```python
from build123d import *

# Parameters (mm, degrees)
F0_R      = 16.890202
F1_DEPTH  = 12.7
F2_R      = 12.7
F3_DEPTH  = 50.8
F5_R      = 16.890202
F6_DEPTH  = 12.7
F7_R      = 3.429
F8_DEPTH  = 12.701
F10_DEPTH = 12.7


with BuildPart() as f1:
    # F0 (on Front) → F1 (new body, symmetric)
    with BuildSketch(Plane.XZ):
        Circle(F0_R)
    extrude(amount=F1_DEPTH, both=True)

    # F2 (on Top) → F3 (join)
    with BuildSketch(Plane.XY):
        Circle(F2_R)
    extrude(amount=F3_DEPTH)

    # F5 (on offset) → F6 (cut)
    with BuildSketch(Plane.XZ.offset(12.7)):
        Circle(F5_R)
    extrude(amount=-F6_DEPTH, mode=Mode.SUBTRACT)

    # F7 (on face) → F8 (cut, through all)
    with BuildSketch(Plane.XZ):
        Circle(F7_R)
    extrude(amount=-F8_DEPTH, mode=Mode.SUBTRACT)

    # F9 (on offset) → F10 (cut, through all)
    with BuildSketch(Plane.XZ.offset(12.7)):
        with BuildLine():
            ThreePointArc((13.434605, 29.257544), (0, 20.560373), (-13.434605, 29.257544))
            Line((-13.434605, 29.257544), (-13.434605, 6.106135))
            Line((-13.434605, 6.106135), (13.446192, 6.106135))
            Line((13.446192, 6.106135), (13.446192, 29.257544))
            Line((13.446192, 29.257544), (13.434605, 29.257544))
        make_face()
    extrude(amount=-F10_DEPTH, mode=Mode.SUBTRACT)


solid = f1.part
```
Source: CAD feature listing. Evaluate the final solid. Frame: model axes, mm. A direction names the side the tool comes from. Give positions to 0.01 mm unless a question says otherwise; leave off trailing zeros. Loops run counter-clockwise (first coordinate to the right, second up) from the corner with the lowest first, then second, coordinate; pieces in that order, holes last. Notation, with made-up numbers: (37.25, -22.75) -> (64.25, -22.75) arc R15 cw to (64.25, -13.75) -> close; hole circle Ø8 at (-30.5, 42). An arc over 180 degrees is marked (long way). Use a Markdown table: item, result. Add a question column.
(1) Section query B-B (z = 2). Output: boundary loops of the cut face in (x, y), then the cut area to 3 significant figures.
(2) Access query for faces 1 (the face through (0.21, -5.03, 20.56)), 2 (the face through (-1.653, 12.592, 35.097)), 3 (the face through (0, 12.7, -4)). Directions: +Z, -Z, +X, -X, +Y, -Y. A direction counts if a zero-diameter tool reaches every point of the face in a straight line with its end or side. Return the directions, or none.
(3) Section query C-C (z = 33.5). Output: boundary loops of the cut face in (x, y).
(4) Ray query, line 1 (Z direction, x = 0, y = 9.5); line 2 (X direction, y = 5.5, z = 0); line 3 (Y direction, x = 5, z = 16). Return the intervals inside material, ascending.
(5) Section query A-A (y = 5.25). Output: boundary loops of the cut face in (x, z).
(6) First-contact query: pin 1 Ø4 at (x, z) = (0, 0) entering from +Y; pin 2 Ø3 at (x, z) = (2, 22.5) entering from +Y; pin 3 Ø4 at (y, z) = (-7.5, 43) entering from -X; pin 4 Ø2 at (x, z) = (11.5, 20.5) entering from -Y. Flat tips, straight axial feed; report the tip coordinate or a pass-through.
(7) Section query D-D (y = -8.5). Output: boundary loops of the cut face in (x, z), then the cut area to 3 significant figures.
Checked values:
| question | item | result |
|---|---|---|
| 1 | outline | (-16.77, 0) -> (-2.79, 0) -> (-2.79, 12.7) -> (-16.77, 12.7) -> close; (2.79, 0) -> (16.77, 0) -> (16.77, 12.7) -> (2.79, 12.7) -> close |
| 1 | area | 355 mm^2 |
| 2 | face 1 | -Z, -Y |
| 2 | face 2 | +Z |
| 2 | face 3 | +Z, -Z, +X, -X, +Y |
| 3 | outline | circle Ø25.4 at (0, 0) |
| 4 | line 1 | -16.89 to -3.43, 3.43 to 50.8 |
| 4 | line 2 | -16.89 to -3.43, 3.43 to 16.89 |
| 4 | line 3 | 0 to 12.7 |
| 5 | outline | (-11.56, 12.31) arc R16.89 ccw (long way) to (11.56, 12.31) -> (11.56, 50.8) -> (-11.56, 50.8) -> close; hole circle Ø6.86 at (0, 0) |
| 6 | pin 1 | through |
| 6 | pin 2 | y = 12.69 |
| 6 | pin 3 | x = -11.45 |
| 6 | pin 4 | y = 0 |
| 7 | outline | (-9.44, 23.98) arc R14.72 ccw to (9.44, 23.98) -> (9.44, 50.8) -> (-9.44, 50.8) -> close |
| 7 | area | 550 mm^2 |
